from build123d import *

# Parameters (mm, degrees)
SKETCH_1_W          = 76.2
SKETCH_1_H          = 30
SKETCH_1_W_2        = 8.9408
SKETCH_1_H_2        = 11.0998
SKETCH_1_W_3        = 12.1539
SKETCH_1_H_3        = 10.7442
EXTRUDE_1_DEPTH     = 3
SKETCH_2_W          = 19.6215
SKETCH_2_H          = 3
CUT_EXTRUDE_1_DEPTH = 3
SKETCH_3_W          = 3
SKETCH_3_H          = 8.89
CUT_EXTRUDE_2_DEPTH = 3
SKETCH_4_W          = 30.7975
SKETCH_4_H          = 3
EXTRUDE_2_DEPTH     = 3
SKETCH_5_R          = 4.98475
CUT_EXTRUDE_3_DEPTH = 3


with BuildPart() as part:
    # 스케치1 → 보스-돌출1 (new body)
    with BuildSketch(Plane.XY):
        Rectangle(SKETCH_1_W, SKETCH_1_H)
        with Locations((12.9343, -2.4623)):
            Rectangle(SKETCH_1_W_2, SKETCH_1_H_2, mode=Mode.SUBTRACT)
        with Locations((-16.98055, -2.6401)):
            Rectangle(SKETCH_1_W_3, SKETCH_1_H_3, mode=Mode.SUBTRACT)
    extrude(amount=EXTRUDE_1_DEPTH)

    # 스케치2 → 컷-돌출1 (cut)
    with BuildSketch(Plane.XY.offset(3)):
        with Locations((-28.28925, -13.5)):
            Rectangle(SKETCH_2_W, SKETCH_2_H)
        with Locations((28.28925, -13.5)):
            Rectangle(SKETCH_2_W, SKETCH_2_H)
    extrude(amount=-CUT_EXTRUDE_1_DEPTH, mode=Mode.SUBTRACT)

    # 스케치3 → 컷-돌출2 (cut)
    with BuildSketch(Plane.XY.offset(3)):
        with Locations((-36.6, 1.5)):
            Rectangle(SKETCH_3_W, SKETCH_3_H)
        with Locations((36.6, 1.5)):
            Rectangle(SKETCH_3_W, SKETCH_3_H)
    extrude(amount=-CUT_EXTRUDE_2_DEPTH, mode=Mode.SUBTRACT)

    # 스케치4 → 보스-돌출2 (add)
    with BuildSketch(Plane.XY.offset(3)):
        with Locations((0, 16.5)):
            Rectangle(SKETCH_4_W, SKETCH_4_H)
    extrude(amount=-EXTRUDE_2_DEPTH)

    # 스케치5 → 컷-돌출3 (cut)
    with BuildSketch(Plane.XY.offset(3)):
        with Locations((28.115, -5.65)):
            Circle(SKETCH_5_R)
    extrude(amount=-CUT_EXTRUDE_3_DEPTH, mode=Mode.SUBTRACT)


solid = part.part
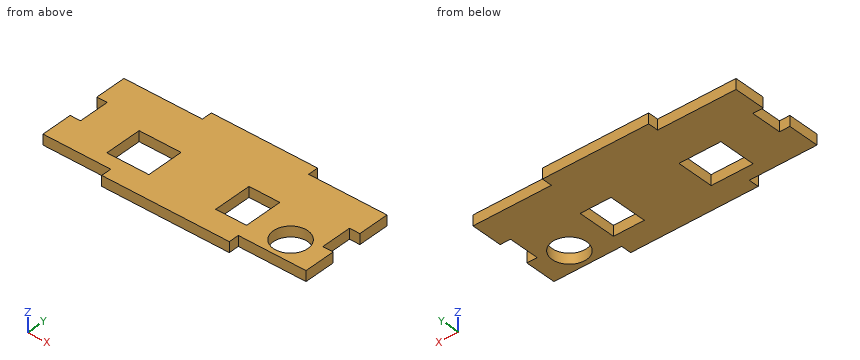
Here's how the part is built. I have some questions about the finished solid (model axes, mm). Round coordinates to 2 decimals unless told otherwise and drop trailing zeros. Loops run counter-clockwise (first coordinate to the right, second up) from the corner with the lowest first, then second, coordinate; pieces in that order, holes last.
1. If I drill on line 1 along Y through (x, z) = (16, 2.4); line 2 along Y through (x, z) = (-15, 1.1); line 3 along X through (y, z) = (2.5, 0.7), over which ranges is the centre line in solid material (lowest first)?
Answer list:
line 1: y = -15 to -8.01, 3.09 to 15
line 2: y = -15 to -8.01, 2.73 to 18
line 3: x = -35.1 to -23.06, -10.9 to 8.46, 17.4 to 35.1
2. If we section it at C-C on y = 4.5: Write out the boundary of the cut face in (x, z).
Answer list:
outline: (-35.1, 0) - (35.1, 0) - (35.1, 3) - (-35.1, 3) - close
3. If we section it at A-A on z = 1.85: Count the separate pieces of the cut face and the enclosed holes in it, plus the area to 3 significant figures.
Answer list:
separate pieces: 1
enclosed holes: 3
area: 1,900 mm2
4. If we section it at B-B on y = -5.65: Write out the boundary of the cut face in (x, z).
Answer list:
outline: (-38.1, 0) - (-23.06, 0) - (-23.06, 3) - (-38.1, 3) - close; (-10.9, 0) - (8.46, 0) - (8.46, 3) - (-10.9, 3) - close; (17.4, 0) - (23.13, 0) - (23.13, 3) - (17.4, 3) - close; (33.1, 0) - (38.1, 0) - (38.1, 3) - (33.1, 3) - close
5. For P1, Ø1.5, axis at x = -19.5, z = 1.5, coming from the -Y side; P2, Ø1.5, axis at y = 16, z = 1, coming from the +X side, each with a flat end and sliding along its axis, tell me the tip position at first contact or that it passes through.
Answer list:
P1: stops at y = -12
P2: stops at x = 15.4
